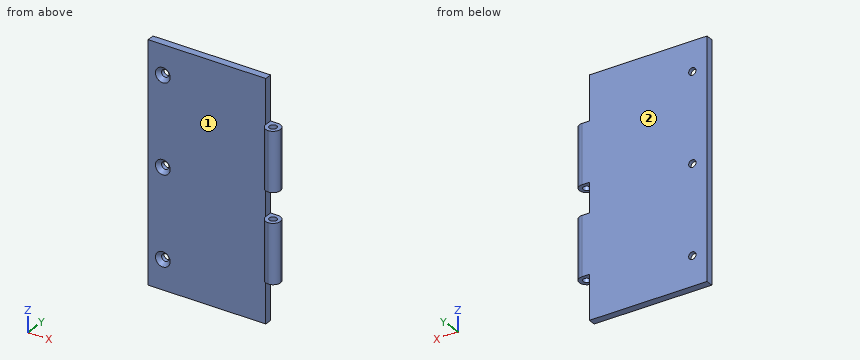
```python
from build123d import *

# Parameters (mm, degrees)
F0_W           = 50.8
F0_H           = 101.6
F1_DEPTH       = 3.175
F2_W           = 6.35
F2_H           = 25.4
F3_DEPTH       = 6.35
F5_DEPTH       = 82.551
F6_R           = 1.5875
F7_DEPTH       = 82.551
F9_D           = 3.175
F9_CSINK_D     = 6.35
F9_CSINK_ANGLE = 90


with BuildPart() as f1:
    # F0 (on Front) → F1 (new body)
    with BuildSketch(Plane.XZ):
        Rectangle(F0_W, F0_H)
    extrude(amount=F1_DEPTH)

    # F2 (on face) → F3 (join)
    with BuildSketch(Plane.YZ.offset(25.4)):
        with Locations((-3.175, 19.05)):
            Rectangle(F2_W, F2_H)
        with Locations((-3.175, -19.05)):
            Rectangle(F2_W, F2_H)
    extrude(amount=F3_DEPTH)

    # F4 (on face) → F5 (cut, through all)
    with BuildSketch(Plane.XY.offset(31.75)):
        with BuildLine():
            Line((31.75, -6.35), (31.75, -3.175))
            ThreePointArc((31.75, -3.175), (30.8200640303, -5.4200640303), (28.575, -6.35))
            Line((28.575, -6.35), (31.75, -6.35))
        make_face()
        with BuildLine():
            ThreePointArc((28.575, 0), (30.8200640303, -0.9299359697), (31.75, -3.175))
            Line((31.75, -3.175), (31.75, 0))
            Line((31.75, 0), (28.575, 0))
        make_face()
        with BuildLine():
            Line((25.4, -6.35), (28.575, -6.35))
            ThreePointArc((28.575, -6.35), (26.3299359697, -5.4200640303), (25.4, -3.175))
            Line((25.4, -3.175), (25.4, -6.35))
        make_face()
    extrude(amount=-F5_DEPTH, mode=Mode.SUBTRACT)

    # F6 (on face) → F7 (cut, through all)
    with BuildSketch(Plane.XY.offset(31.75)):
        with Locations((28.575, -3.175)):
            Circle(F6_R)
    extrude(amount=-F7_DEPTH, mode=Mode.SUBTRACT)

    # F9 (through all)
    with Locations(Plane.XZ.offset(3.175)):
        with Locations((-19.05, 38.1), (-19.05, 0), (-19.05, -38.1)):
            CounterSinkHole(F9_D / 2, F9_CSINK_D / 2, counter_sink_angle=F9_CSINK_ANGLE)


solid = f1.part
```
Geometry check sheet. Reference: the model listing, model coordinates, mm. Face numbers are marked on the shaded views. A direction names the side the tool comes from. Give positions to 0.01 mm unless a question says otherwise; leave off trailing zeros. Loops run counter-clockwise (first coordinate to the right, second up) from the corner with the lowest first, then second, coordinate; pieces in that order, holes last. Notation, with made-up numbers: M 74.25,-22.75 L 91.25,-22.75 A27 cw 91.25,-0.75 Z; hole C 67,69.5 d10. An arc over 180 degrees is marked long. Write item = value, one per line. Start each with the question number.
1. Section check B-B, the plane z = 0. Enter the section's corners in (x, y) (1 decimal).
2. Section check A-A, the plane x = -19.05. Enter the section's corners in (y, z) (1 decimal).
3. Thickness scan on probe 1 along X at (y, z) = (-1.25, 38.1); probe 2 along Z at (x, y) = (-20, -1.75); probe 3 along Y at (x, z) = (20, 34) (3 decimals). Record the ranges inside material, lowest first.
4. Go/stop test with flat-tipped pins: P1, Ø1.6, axis at y = -1.5, z = 43, coming from the +X side; P2, Ø1.9, axis at x = 30, y = -4, coming from the -Z side; P3, Ø1, axis at x = 18, z = 15, coming from the -Y side (3 decimals); P4, Ø1.9, axis at x = -19.05, z = -38.1, coming from the -Y side. Record where each tip stops, or that it passes through.
5. Tool access check on the marked faces 1 and 2. Record the directions out of +Z, -Z, +X, -X, +Y, -Y that give a thin tool (end or side, any length) a straight path to the whole face; none if there is none.
6. Section check D-D, the plane x = 12. Enter the section's corners in (y, z) (3 decimals), plus the area to 3 significant figures.
Values follow:
q1.outline = M -25.4,-3.2 L -22.2,-3.2 L -20.6,-1.6 L -20.6,0 L -25.4,0 Z; M -17.5,-1.6 L -15.9,-3.2 L 25.4,-3.2 L 25.4,0 L -17.5,0 Z
q2.outline = M -3.2,-50.8 L 0,-50.8 L 0,-39.7 L -1.6,-39.7 L -3.2,-41.3 Z; M -3.2,-34.9 L -1.6,-36.5 L 0,-36.5 L 0,-1.6 L -1.6,-1.6 L -3.2,-3.2 Z; M -3.2,3.2 L -1.6,1.6 L 0,1.6 L 0,36.5 L -1.6,36.5 L -3.2,34.9 Z; M -3.2,41.3 L -1.6,39.7 L 0,39.7 L 0,50.8 L -3.2,50.8 Z
q3.probe_1 = -25.4 to -20.64, -17.46 to 25.4
q3.probe_2 = -50.8 to -39.57, -36.63 to -1.47, 1.47 to 36.63, 39.57 to 50.8
q3.probe_3 = -3.175 to 0
q4.P1 = 25.4
q4.P2 = -31.75
q4.P3 = -3.175
q4.P4 = through
q5.face_1 = +Z, -Z, -X, -Y
q5.face_2 = +Z, -Z, +X, -X, +Y
q6.outline = M -3.175,-50.8 L 0,-50.8 L 0,50.8 L -3.175,50.8 Z
q6.area = 323 mm^2
